Autodesk Inventor part; units mm, degrees
ref_plane "Work Plane1" through (59.6, 59.6, 0) normal (0.7071, -0.7071, 0) x (0, 0, -1)
ref_plane "YZ Plane" through (0, 0, 0) normal (1, 0, 0) x (0, 1, 0)
ref_plane "XZ Plane" through (0, 0, 0) normal (0, 1, 0) x (-1, 0, 0)
sketch "Sketch1" plane through (0, 0, 0) normal (0, 0, 1) x (1, 0, 0)
  line L0 (-59.6, 59.6) -> (59.6, 59.6)
  line L1 (59.6, 59.6) -> (59.6, -59.6)
  line L2 (59.6, -59.6) -> (-59.6, -59.6)
  line L3 (-59.6, -59.6) -> (-59.6, 59.6)
  point P0 (0, 0)
  point P1 (59.6, 0)
  point P2 (0, 59.6)
  dimension "d0" = 119.2
extrude "Extrusion1" add sketch "Sketch1" along normal blind 38.3
fillet "Fillet1" radius 5 4 edges at (-59.6, 59.6, 19.15) (59.6, 59.6, 19.15) (59.6, -59.6, 19.15) (-59.6, -59.6, 19.15)
sketch "Sketch2" plane through (0, 0, 38.3) normal (0, 0, 1) x (1, 0, 0)
  circle A0 centre (52.6, 52.6) radius 1.75
  line L0 (54.6, 59.6) -> (-54.6, 59.6)
  line L1 (59.6, -54.6) -> (59.6, 54.6)
  point P0 (0, 0)
  dimension "d4" = 7
  dimension "d5" = 7
  dimension "d6" = 3.5
extrude "Extrusion2" cut sketch "Sketch2" against normal through all
mirror "Mirror1" about plane through (0, 0, 0) normal (1, 0, 0) of "Extrusion2"
mirror "Mirror2" about plane through (0, 0, 0) normal (0, 1, 0) of "Extrusion2", "Mirror1"
ref_plane "Work Plane1" through (59.6, 59.6, 0) normal (0.7071, -0.7071, 0) x (0, 0, -1)
sketch "Sketch3" plane through (59.6, 59.6, 0) normal (0.7071, -0.7071, 0) x (0, 0, -1)
  line L0 (-32.3, -14.0711) -> (-6, -14.0711)
  line L1 (-6, -14.0711) -> (-6, 12.5661)
  line L2 (-6, 12.5661) -> (-32.3, 12.5661)
  line L3 (-32.3, 12.5661) -> (-32.3, -14.0711)
  line L4 (-38.3, -3.5355) -> (-38.3, -2.0711)
  line L5 (0, -2.0711) -> (-38.3, -2.0711) construction
  line L6 (-38.3, -3.5355) -> (-38.3, -80.7516)
  line L7 (0, -3.5355) -> (0, -80.7516)
  point P0 (0, -84.2871)
  dimension "d9" = 12
  dimension "d10" = 6
  dimension "d11" = 6
extrude "Extrusion3" cut sketch "Sketch3" along normal through all both and the other way through all
mirror "Mirror3" about plane through (0, 0, 0) normal (1, 0, 0) of "Extrusion3"
mirror "Mirror4" about plane through (0, 0, 0) normal (0, 1, 0) of "Extrusion3", "Mirror3"
sketch "Sketch4" plane through (0, 0, 38.3) normal (0, 0, 1) x (1, 0, 0)
  circle A0 centre (0, 0) radius 56.75
  dimension "d14" = 113.5
extrude "Extrusion4" cut sketch "Sketch4" against normal through all
properties part number "AC-fan-case"
Geometry: final body of the model. Coordinates: model frame, mm. A direction names the side the tool comes from. Coordinates: 2 decimals unless noted, no trailing zeros. Order: outer loops, then holes, each group sorted by start corner. A loop starts at its lowest first (then second) coordinate and runs counter-clockwise, first axis right, second up. Notation, with made-up numbers: M 28,-19 L 87,-19 A13 ccw 87,-1 Z; hole C 41,58.5 d7. An arc over 180 degrees is marked long. Answer as CSV lines item,"result".
Q1. Set-up query: faces 1 (the flat face through (-54, 54, 6)), 2 (the cylindrical face through (52.22, 50.89, 3.04)), 3 (the flat face through (54, -54, 6)), 4 (the flat face through (49.5, 49.8, 19.3)), 5 (the flat face through (-49.5, -49.8, 19.3)). Return all of +Z, -Z, +X, -X, +Y, -Y with unobstructed straight access to the full face (end or side cutting, diameter ignored); none if empty.
Answers:
face 1,"-X, +Y"
face 2,"+Z, -Z"
face 3,"+X, -Y"
face 4,"+X, +Y"
face 5,"-X, -Y"
Q2. Section C-C on z = 29.5. Return the cut outline in (x, y).
Answers:
outline,"M -59.6,-39.7 L -39.7,-59.6 L 39.7,-59.6 L 59.6,-39.7 L 59.6,39.7 L 39.7,59.6 L -39.7,59.6 L -59.6,39.7 Z; hole C 0,0 d113.5"
Q3. Section D-D on x = 52.6. Count the separate pieces of the cut face and the enclosed holes in it, and give its area (3 significant figures).
Answers:
separate pieces,"6"
enclosed holes,"0"
area,"2,170 mm^2"
Q4. Draft query along Z for faces 6 (the flat face through (54, 54, 6)), 7 (the flat face through (-35.6, 44.4, 38.3)), 8 (the cylindrical face through (-58.17, -58.1, 3.04)). Return one class per face: pulls with the +Z half, pulls with the -Z half, needs draft (parallel to the pull), parting line crosses it, or undercut.
Answers:
face 6,"undercut"
face 7,"pulls with the +Z half"
face 8,"needs draft"
Q5. First-contact query: P1, Ø3, axis at x = -52.6, y = 52.6, coming from the +Z side; P2, Ø3, axis at x = -47, z = 20.5, coming from the -Y side. Flat tips, straight axial feed; report the tip coordinate or a pass-through.
Answers:
P1,"passes through"
P2,"stops at y = -53.8"
Q6. Section A-A on x = 0. Return the cut outline in (y, z), and give its area (3 significant figures).
Answers:
outline,"M -59.6,0 L -56.75,0 L -56.75,38.3 L -59.6,38.3 Z; M 56.75,0 L 59.6,0 L 59.6,38.3 L 56.75,38.3 Z"
area,"218 mm^2"
Q7. Line query: probe 1 along Y at (x, z) = (1, 31); probe 2 along Z at (x, y) = (53, 48.5); probe 3 along X at (y, z) = (-52, 1). Output: solid intervals per line, ascending. Write a range as [from, to].
Answers:
probe 1,"y = [-59.6, -56.74], [56.74, 59.6]"
probe 2,"z = [0, 6], [32.3, 38.3]"
probe 3,"x = [-59.6, -54.24], [-50.96, -22.73], [22.73, 50.96], [54.24, 59.6]"
